Model file for the job. Use its own axes, mm. A direction names the side the tool comes from. Coordinates: 2 decimals unless noted, no trailing zeros. Write each loop counter-clockwise with the first axis right and the second up, starting at its lowest first coordinate (ties: lowest second). Pieces come first, ordered by that corner, then holes. Notation, with made-up numbers: M 26.25,20.5 L 45.25,20.5 A19 ccw 45.25,33.5 Z; hole C 39,58.25 d5. An arc over 180 degrees is marked long. One line per question, with ' | ' between items. Start each with the question number.
(1) Wall check: probe 1 along X at (y, z) = (28.75, 0.2); probe 2 along X at (y, z) = (27.5, 2.15); probe 3 along Y at (x, z) = (52.5, 2.8). Give the ranges that are in metal, low to high.
(2) Cut at D-D (z = 0.55). Write the cut outline in (x, y).
(3) Cut at B-B (x = 61). Write the cut outline in (y, z), plus the area to 3 significant figures.
(4) Flat gauge pins, fed straight in: pin 1 Ø1.5 at (y, z) = (27, 2.5) entering from -X; pin 2 Ø1 at (y, z) = (31.5, 2.5) entering from +X; pin 3 Ø1.5 at (x, z) = (43.5, 1) entering from +Y. Where does each tip first touch, or does it go through?
(5) Cut at C-C (y = 31.5). Write the cut outline in (x, z), plus the area to 3 significant figures.
(6) Two-plate mould, pull along X, no slides. Class faces 1 (the face through (65.116, 28.988, 1.479)), 2 (the face through (46, 29, 3)): +X half, -X half, draft (parallel to the pull), parting line (faces both ways), or undercut.
(7) Cut at A-A (y = 29.25). Write the cut outline in (x, z), plus the area to 3 significant figures.
(8) Tool access for faces 3 (the face through (29.43, 29.78, 1.48)), 4 (the face through (46, 30.363, 1)), 5 (the face through (58.354, 27.242, 1.521)): list every direction of +Z, -Z, +X, -X, +Y, -Y with a clear straight run to the whole face (end or side of a thin tool).
Autodesk Fusion 360 part; units mm, degrees
sketch "Sketch1" plane through (0, 0, 0) normal (0, 0, 1) x (1, 0, 0)
  circle A0 centre (30.6182, 28.8633) radius 1.5
  circle A1 centre (30.6182, 28.8633) radius 3.5
  circle A2 centre (61.6182, 28.8633) radius 1.5
  circle A3 centre (61.6182, 28.8633) radius 3.5
  line L0 (30.6182, 28.8633) -> (61.6182, 28.8633)
  line L1 (33.7805, 30.3633) -> (59, 30.3633)
  line L2 (33.7805, 27.3633) -> (59, 27.3633)
  dimension "d1" = 3
  dimension "d2" = 7
  dimension "d3" = 3
  dimension "d4" = 7
  dimension "d5" = 31
  dimension "d6" = 1.5
extrude "Extrude1" add sketch "Sketch1" along normal blind 3
fillet "Fillet1" radius 1 4 edges at (33.7805, 30.3633, 1.5) (58.456, 30.3633, 1.5) (33.7805, 27.3633, 1.5) (58.456, 27.3633, 1.5)
Filled in:
1) probe 1: 27.12 to 29.12, 32.11 to 60.12, 63.11 to 65.12 | probe 2: 27.39 to 29.99, 31.24 to 60.99, 62.24 to 64.84 | probe 3: 27.36 to 30.36
2) outline: M 33.53,26.92 A1 cw 34.36,27.36 L 57.88,27.36 A1 cw 58.71,26.92 A3.5 ccw long 58.71,30.81 A1 cw 57.88,30.36 L 34.36,30.36 A1 cw 33.53,30.81 A3.5 ccw long Z; hole C 30.62,28.86 d3; hole C 61.62,28.86 d3
3) outline: M 25.42,0 L 27.5,0 L 27.5,3 L 25.42,3 Z; M 30.23,0 L 32.31,0 L 32.31,3 L 30.23,3 Z | area: 12.5 mm²
4) pin 1: x = 27.3 | pin 2: x = 64.39 | pin 3: y = 30.36
5) outline: M 28.32,0 L 32.92,0 L 32.92,3 L 28.32,3 Z; M 59.32,0 L 63.92,0 L 63.92,3 L 59.32,3 Z | area: 27.6 mm²
6) face 1: undercut | face 2: draft
7) outline: M 27.14,0 L 29.17,0 L 29.17,3 L 27.14,3 Z; M 32.07,0 L 60.17,0 L 60.17,3 L 32.07,3 Z; M 63.07,0 L 65.1,0 L 65.1,3 L 63.07,3 Z | area: 96.5 mm²
8) face 3: +Z, -Z | face 4: +Z, -Z, +Y | face 5: +Z, -Z, -Y
